Could you check a few things on this drawing? It's one solid part, dimensions in mm from its lowest x, y, z. A direction names the side the tool comes from. Give positions to 0.01 mm unless a question says otherwise; leave off trailing zeros. Loops run counter-clockwise (first coordinate to the right, second up) from the corner with the lowest first, then second, coordinate; pieces in that order, holes last. Notation, with made-up numbers: (-22, -12.75) - (22, -12.75) arc R37 ccw to (22, 25.25) - close; hole circle Ø9 at (-32.5, 68). An arc over 180 degrees is marked (long way). Answer as a JSON object with one key per item and string values.
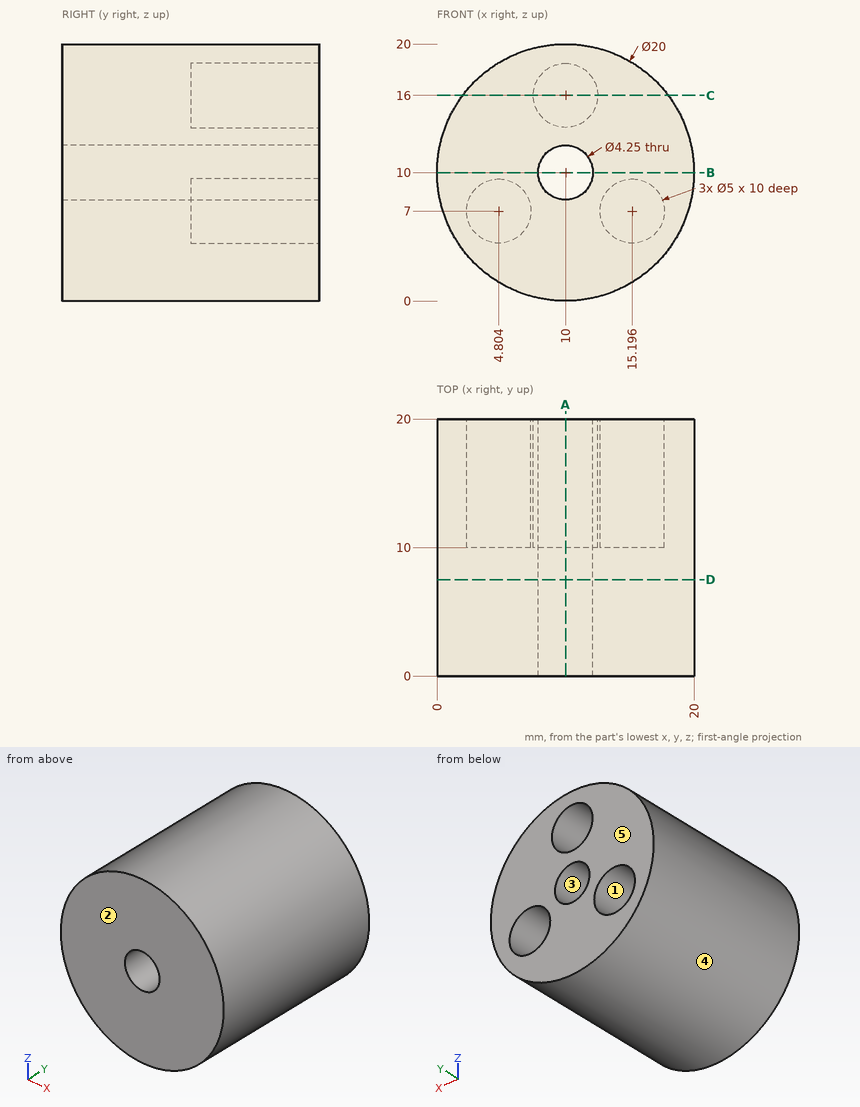
1) Imagine slicing it at A-A on x = 10. Write out the boundary of the cut face in (y, z) (3 decimals), and give its area (3 significant figures).
Check sheet entries:
{"outline": "(0, 0) - (20, 0) - (20, 7.875) - (0, 7.875) - close; (0, 12.125) - (20, 12.125) - (20, 13.5) - (10, 13.5) - (10, 18.5) - (20, 18.5) - (20, 20) - (0, 20) - close", "area": "265 mm2"}
2) Which directions (+Z, -Z, +X, -X, +Y, -Y) give clear straight access to the entire face, cutting with the end or side of a thin tool? Please do the marked faces 1 and 2.
Check sheet entries:
{"face 1": "+Y", "face 2": "+Z, -Z, +X, -X, -Y"}
3) I'm going to push flat-ended pins straight in: P1, Ø1.5, axis at x = 11.5, y = 7.5, coming from the +Z side; P2, Ø2.5, axis at x = 4, z = 7.5, coming from the +Y side; P3, Ø3, axis at y = 15, z = 15.5, coming from the -X side (1 decimal). Where does each tip first touch, or does it pass through?
Check sheet entries:
{"P1": "z = 19.97", "P2": "y = 10", "P3": "x = 0.8"}
4) Imagine slicing it at C-C on z = 16. Write out the boundary of the cut face in (x, y), and give its area (3 significant figures).
Check sheet entries:
{"outline": "(2, 0) - (18, 0) - (18, 20) - (12.5, 20) - (12.5, 10) - (7.5, 10) - (7.5, 20) - (2, 20) - close", "area": "270 mm2"}
5) Imagine slicing it at D-D on y = 7.5. Write out the boundary of the cut face in (x, z) (3 decimals).
Check sheet entries:
{"outline": "circle Ø20 at (10, 10); hole circle Ø4.25 at (10, 10)"}
6) I need wall thicknesses on L1, parallel to X at y = 17.5, z = 10 (3 decimals); L2, parallel to X at y = 14, z = 7; L3, parallel to X at y = 12, z = 6 (1 decimal). Which ranges of each line are inside material? Lowest first, please.
Check sheet entries:
{"L1": "0 to 7.875, 12.125 to 20", "L2": "0.46 to 2.3, 7.3 to 12.7, 17.7 to 19.54", "L3": "0.8 to 2.5, 7.1 to 12.9, 17.5 to 19.2"}
7) Imagine slicing it at B-B on z = 10. Write out the boundary of the cut face in (x, y) (3 decimals), and give its area (3 significant figures).
Check sheet entries:
{"outline": "(0, 0) - (7.875, 0) - (7.875, 20) - (0, 20) - close; (12.125, 0) - (20, 0) - (20, 20) - (12.125, 20) - close", "area": "315 mm2"}
8) If we mould it in two halves opening along Z, with no side actions, what happens to the marked faces 3, 4 and 5? For each: released by +Z, released by -Z, zero draft, split by the parting line, or undercut.
Check sheet entries:
{"face 3": "undercut", "face 4": "split by the parting line", "face 5": "zero draft"}
